from build123d import *

# Parameters (mm, degrees)
BOSS_EXTRUDE1_DEPTH = 10
BOSS_EXTRUDE2_START = 29.60383513
BOSS_EXTRUDE2_DEPTH = 31.225392193


# Read off the part's stored shape, not the designer's step: Boss-Extrude2
with BuildPart() as part:
    # Sketch1 → Boss-Extrude1 (new body)
    with BuildSketch(Plane(origin=(0, 0, 0), x_dir=(1, 0, 0), z_dir=(0, 1, 0))):
        Polygon((10, 0), (10, 10), (0, 10), (37.469962049, 55.82661754), (62.28046579, 38.961300937), (54.526318582, 27.55420418), (80.350242243, 10), (70, 10), (70, 0), (50, 0), (50, 10), (30, 10), (30, 0), align=None)
    extrude(amount=BOSS_EXTRUDE1_DEPTH)

    # Boss-Extrude2 outline → Boss-Extrude2 (add)
    with BuildSketch(Plane(origin=(0, 0, 0), x_dir=(0.562177220107601, 0, -0.8270167913604233), z_dir=(0.8270167913604233, 0, 0.5621772201076011)).offset(BOSS_EXTRUDE2_START)):
        Polygon((53.441243733, 0), (58.207083275, 10), (53.441243733, 10), align=None)
    extrude(amount=BOSS_EXTRUDE2_DEPTH)


solid = part.part
Design review of the part built by this model. Coordinates are the model's own, in mm. A direction names the side the tool comes from. Round coordinates to 2 decimals unless told otherwise and drop trailing zeros. Loops run counter-clockwise (first coordinate to the right, second up) from the corner with the lowest first, then second, coordinate; pieces in that order, holes last. Notation, with made-up numbers: (55, 30) - (82, 30) arc R17 ccw to (82, 49) - close; hole circle Ø6 at (52.25, -34). An arc over 180 degrees is marked (long way). One line per question, with ' | ' between items.
1. Draft analysis for pull direction Z (two halves, no side actions). For faces 1 (the face through (68.58, 4.93, -20.84)), 2 (the face through (41, 10, -25)), 3 (the face through (40, 5, -10)), 4 (the face through (59.319, 4.93, -34.605)), state which applies: released by +Z, released by -Z, zero draft, split by the parting line, or undercut.
Results are:
face 1: undercut | face 2: zero draft | face 3: released by +Z | face 4: undercut
2. For faces 5 (the face through (70, 5, -5)), 6 (the face through (50, 5, -5)), 7 (the face through (10, 5, -5)), list the 3-axis set-ups (+Z, -Z, +X, -X, +Y, -Y) from which the entire face can be reached by the end or side of a thin tool; tool diameter is ignored.
Results are:
face 5: +Z, +X, +Y, -Y | face 6: +Z, +Y, -Y | face 7: +Z, -X, +Y, -Y
3. We need section D-D, the plane y = 3.25. State the section outline as (x, z) points.
Results are:
outline: (0, -10) - (37.47, -55.83) - (62.28, -38.96) - (55.4, -28.84) - (81.22, -11.28) - (80.35, -10) - (70, -10) - (70, 0) - (50, 0) - (50, -10) - (30, -10) - (30, 0) - (10, 0) - (10, -10) - close
4. Clearance check with flat-ended pins moving along their axes: P1, Ø5, axis at x = 74.5, y = 4.5, coming from the +Z side; P2, Ø1.5, axis at x = 64.5, y = 1.5, coming from the -Z side; P3, Ø5, axis at y = 9, z = -31.5, coming from the +X side; P4, Ø5, axis at x = 56, z = -49, coming from the -Y side. State where each tip first meets the part, or that it passes through.
Results are:
P1: stops at z = -10 | P2: stops at z = -22.31 | P3: stops at x = 60.57 | P4: passes through
5. We need section B-B, the plane x = 17.5. State the section outline as (y, z) points, and give its area (3 significant figures).
Results are:
outline: (0, -31.4) - (10, -31.4) - (10, 0) - (0, 0) - close | area: 314 mm²
6. We need section C-C, the plane z = -49. State the section outline as (x, y) points, and give its area (3 significant figures).
Results are:
outline: (31.89, 0) - (47.51, 0) - (47.51, 10) - (31.89, 10) - close | area: 156 mm²
7. We need section A-A, the plane y = 8.5. State the section outline as (x, z) points, and give its area (3 significant figures).
Results are:
outline: (0, -10) - (37.47, -55.83) - (62.28, -38.96) - (56.8, -30.9) - (82.63, -13.35) - (80.35, -10) - (70, -10) - (70, 0) - (50, 0) - (50, -10) - (30, -10) - (30, 0) - (10, 0) - (10, -10) - close | area: 2,360 mm²
8. For L1, parallel to X at y = 7.25, z = -6.5; L2, parallel to X at y = 7.5, z = -18.5; L3, parallel to X at y = 1.75, z = -31.5, list the stretches that pass through material, from the lowest coordinate up. Write a range as [from, to].
Results are:
L1: x = [10, 30], [50, 70] | L2: x = [6.95, 74.2] | L3: x = [17.58, 57.21]
